For this review, take the finished solid that the model builds, in its own axes (mm). A direction names the side the tool comes from. Coordinates: 2 decimals unless noted, no trailing zeros. Loops run counter-clockwise (first coordinate to the right, second up) from the corner with the lowest first, then second, coordinate; pieces in that order, holes last. Notation, with made-up numbers: (-26, 46.5) -> (-14, 46.5) arc R17 ccw to (-14, 62.5) -> close; hole circle Ø5 at (38.25, 45.5). An arc over 180 degrees is marked (long way). Answer in a Markdown table with one row per item.
from build123d import *

# Parameters (mm, degrees)
F1_DEPTH  = 400
F2_R      = 100
F3_R      = 100
F4_R      = 100
F5_SIZE   = 50
F6_SIZE   = 50
F7_R      = 50
F8_DEPTH  = 25.4
F8_FACE_R = 50
F9_DEPTH  = 425.401
F10_R     = 25
F11_DEPTH = 600.001


with BuildPart() as f1:
    # F0 (on Front) → F1 (new body)
    with BuildSketch(Plane.XZ):
        Polygon((-480.112339, 99.865262), (-480.112339, -100.134738), (419.887661, -100.134738), (419.887661, 499.865262), (119.887661, 499.865262), (119.887661, 299.865262), (-180.112339, 299.865262), (-180.112339, 99.865262), align=None)
    extrude(amount=F1_DEPTH)

    # F2
    f2_edges = [f1.edges().sort_by_distance(p)[0] for p in [
        (-330.112339, 0, 99.865262),
        (-330.112339, -400, 99.865262),
        (-480.112339, -200, 99.865262),
    ]]
    fillet(f2_edges, radius=F2_R)

    # F3
    f3_edges = [f1.edges().sort_by_distance(p)[0] for p in [
        (-30.112339, 0, 299.865262),
        (-180.112339, -200, 299.865262),
        (-30.112339, -400, 299.865262),
    ]]
    fillet(f3_edges, radius=F3_R)

    # F4
    f4_edges = [f1.edges().sort_by_distance(p)[0] for p in [
        (269.887661, 0, 499.865262),
        (119.887661, -200, 499.865262),
        (269.887661, -400, 499.865262),
    ]]
    fillet(f4_edges, radius=F4_R)

    # F5
    f5_edges = [f1.edges().sort_by_distance(p)[0] for p in [
        (419.887661, -400, 149.865262),
        (419.887661, -200, -100.134738),
    ]]
    chamfer(f5_edges, length=F5_SIZE)

    # F6
    f6_edges = [f1.edges().sort_by_distance(p)[0] for p in [
        (-55.112339, -400, -100.134738),
        (-480.112339, -200, -100.134738),
        (-55.112339, 0, -100.134738),
    ]]
    chamfer(f6_edges, length=F6_SIZE)

    # F7 (on face) → F8 (join)
    with BuildSketch(Plane.XZ.offset(400)):
        with Locations((244.887661, -0.134738)):
            Circle(F7_R)
    extrude(amount=F8_DEPTH)

    # F8_face (on face) → F9 (cut, through all)
    with BuildSketch(Plane(origin=(244.887661, -425.4, -0.134738), x_dir=(1, 0, 0), z_dir=(0, -1, 0))):
        Circle(F8_FACE_R)
    extrude(amount=-F9_DEPTH, mode=Mode.SUBTRACT)

    # F10 (on face) → F11 (cut, through all)
    with BuildSketch(Plane.XY.offset(499.865262)):
        with Locations((292.502016, -203.040093)):
            Circle(F10_R)
        with Locations((15.382883, -205.770329)):
            Circle(F10_R)
        with Locations((-283.578157, -200.309843)):
            Circle(F10_R)
    extrude(amount=-F11_DEPTH, mode=Mode.SUBTRACT)


solid = f1.part
Item 1: The part is to be moulded in two halves that separate along X. For faces 1 (the cylindrical face through (12, -181, 103)), 2 (the cylindrical face through (-260.485, -209.885, 1.265)), 3 (the flat face through (-36, -198, -100.135)), 4 (the cylindrical face through (-162.65, -202.8, 256.32)), say which applies: +X half, -X half, draft (parallel to the pull), parting line (faces both ways), or undercut.
Worked answers:
| item | result |
|---|---|
| face 1 | undercut |
| face 2 | undercut |
| face 3 | draft |
| face 4 | -X half |
Item 2: Take a section at A-A, the plane z = -32. State the section outline as (x, y) points, and give its area (3 significant figures).
Worked answers:
| item | result |
|---|---|
| outline | (-480.11, -400) -> (206.36, -400) -> (206.36, 0) -> (-480.11, 0) -> close; (283.42, -400) -> (369.89, -400) -> (419.89, -350) -> (419.89, -50) -> (369.89, 0) -> (283.42, 0) -> (283.42, -179.75) arc R25 cw (long way) to (283.42, -226.33) -> close; hole circle Ø50 at (-283.58, -200.31); hole circle Ø50 at (15.38, -205.77) |
| area | 321,000 mm² |
Item 3: For L1, parallel to X at y = -200, z = 301; L2, parallel to Z at x = 282, y = -293; L3, parallel to X at y = -221, z = 465, list the stretches that pass through material, from the lowest coordinate up.
Worked answers:
| item | result |
|---|---|
| L1 | 119.89 to 267.69, 317.32 to 419.89 |
| L2 | -100.13 to -33.64, 33.37 to 499.87 |
| L3 | 144.01 to 275.11, 309.89 to 404.75 |
Item 4: Insertion check: pin 1 (3 mm diameter, centred on y = -137.5, z = 180.5, fed in from -X); pin 2 (6 mm diameter, centred on x = -282.5, y = -308.5, fed in from +Z); pin 3 (6 mm diameter, centred on y = -258.5, z = 279.5, fed in from -X) (3 decimals). Each pin has a flat end and moves straight along its axis. Give the tip position at first contact, or say it passes through.
Worked answers:
| item | result |
|---|---|
| pin 1 | x = -180.11 |
| pin 2 | z = 99.71 |
| pin 3 | x = -144.355 |
Item 5: Take a section at B-B, the plane y = -136. State the section outline as (x, z) points, and give its area (3 significant figures).
Worked answers:
| item | result |
|---|---|
| outline | (-480.11, -50.13) -> (-430.11, -100.13) -> (369.89, -100.13) -> (419.89, -50.13) -> (419.89, 449.87) -> (369.89, 499.87) -> (219.89, 499.87) arc R100 ccw to (119.89, 399.87) -> (119.89, 299.87) -> (-80.11, 299.87) arc R100 ccw to (-180.11, 199.87) -> (-180.11, 99.87) -> (-380.11, 99.87) arc R100 ccw to (-480.11, -0.13) -> close; hole circle Ø100 at (244.89, -0.13) |
| area | 342,000 mm² |
Item 6: Take a section at C-C, the plane x = 96. State the section outline as (y, z) points.
Worked answers:
| item | result |
|---|---|
| outline | (-400, -50.13) -> (-350, -100.13) -> (-50, -100.13) -> (0, -50.13) -> (0, 199.87) arc R100 ccw to (-100, 299.87) -> (-300, 299.87) arc R100 ccw to (-400, 199.87) -> close |
Item 7: Take a section at D-D, the plane z = 386.5. State the section outline as (x, y) points.
Worked answers:
| item | result |
|---|---|
| outline | (119.89, -400) -> (369.89, -400) -> (419.89, -350) -> (419.89, -50) -> (369.89, 0) -> (119.89, 0) -> close; hole circle Ø50 at (292.5, -203.04) |
Item 8: For faces 5 (the flat face through (21, -176, 299.865)), 6 (the flat face through (296, -176, 499.865)), list the 3-axis set-ups (+Z, -Z, +X, -X, +Y, -Y) from which the entire face can be reached by the end or side of a thin tool; tool diameter is ignored.
Worked answers:
| item | result |
|---|---|
| face 5 | +Z, -X, +Y, -Y |
| face 6 | +Z, +X, -X, +Y, -Y |
